from build123d import *

# Parameters (mm, degrees)
SKETCH1_R           = 32.5
BOSS_EXTRUDE1_DEPTH = 3
BOSS_EXTRUDE6_DEPTH = 3
CUT_EXTRUDE1_DEPTH  = 3
SKETCH5_R           = 7
BOSS_EXTRUDE7_DEPTH = 3
SKETCH7_R           = 1.9
CUT_EXTRUDE2_DEPTH  = 3


with BuildPart() as part:
    # Sketch1 → Boss-Extrude1 (new body)
    with BuildSketch(Plane.XY):
        Circle(SKETCH1_R)
    extrude(amount=BOSS_EXTRUDE1_DEPTH)

    # Sketch2 → Boss-Extrude6 (add)
    with BuildSketch(Plane.XY.offset(3)):
        Polygon((-0.480921932, 36), (-2.2, 32.425452965), (2.2, 32.425452965), (0.480921932, 36), align=None)
        Polygon((6.106641727, 35.481547496), (7.245372738, 31.682086009), (2.899544039, 32.370397655), (5.156639756, 35.632013027), align=None)
        Polygon((11.581995735, 34.089421537), (12.112340352, 30.158600949), (7.927691681, 31.518275724), (10.66722786, 34.386647637), align=None)
        Polygon((16.77216257, 31.857900882), (16.681061949, 27.892511042), (12.760633243, 29.890069241), (15.915153411, 32.294568859), align=None)
        Polygon((21.549343099, 28.841932978), (20.839040439, 24.939614944), (17.279365664, 27.525870054), (20.771195066, 29.407290617), align=None)
        Polygon((25.795907282, 25.115780963), (24.483892593, 21.372622756), (21.372622756, 24.483892593), (25.115780963, 25.795907282), align=None)
        Polygon((29.407290617, 20.771195066), (27.525870054, 17.279365664), (24.939614944, 20.83904044), (28.841932978, 21.549343099), align=None)
        Polygon((32.294568859, 15.915153411), (29.890069241, 12.760633243), (27.892511042, 16.681061949), (31.857900882, 16.77216257), align=None)
        Polygon((34.386647637, 10.66722786), (31.518275724, 7.927691681), (30.158600949, 12.112340352), (34.089421537, 11.581995735), align=None)
        Polygon((35.632013027, 5.156639756), (32.370397655, 2.899544039), (31.682086009, 7.245372738), (35.481547496, 6.106641727), align=None)
        Polygon((36, -0.480921932), (32.425452965, -2.2), (32.425452965, 2.2), (36, 0.480921932), align=None)
        Polygon((35.481547496, -6.106641727), (31.682086009, -7.245372738), (32.370397655, -2.899544039), (35.632013027, -5.156639756), align=None)
        Polygon((34.089421537, -11.581995735), (30.158600949, -12.112340352), (31.518275724, -7.927691681), (34.386647637, -10.66722786), align=None)
        Polygon((31.857900882, -16.77216257), (27.892511042, -16.681061949), (29.890069241, -12.760633243), (32.294568859, -15.915153411), align=None)
        Polygon((28.841932978, -21.549343099), (24.939614944, -20.839040439), (27.525870054, -17.279365664), (29.407290617, -20.771195066), align=None)
        Polygon((25.115780963, -25.795907282), (21.372622756, -24.483892593), (24.483892593, -21.372622756), (25.795907282, -25.115780963), align=None)
        Polygon((20.771195066, -29.407290617), (17.279365664, -27.525870054), (20.83904044, -24.939614944), (21.549343099, -28.841932978), align=None)
        Polygon((15.915153411, -32.294568859), (12.760633243, -29.890069241), (16.681061949, -27.892511042), (16.77216257, -31.857900882), align=None)
        Polygon((10.66722786, -34.386647637), (7.927691681, -31.518275724), (12.112340352, -30.158600949), (11.581995735, -34.089421537), align=None)
        Polygon((5.156639756, -35.632013027), (2.899544039, -32.370397655), (7.245372738, -31.682086009), (6.106641727, -35.481547496), align=None)
        Polygon((-0.480921932, -36), (-2.2, -32.425452965), (2.2, -32.425452965), (0.480921932, -36), align=None)
        Polygon((-6.106641727, -35.481547496), (-7.245372738, -31.682086009), (-2.899544039, -32.370397655), (-5.156639756, -35.632013027), align=None)
        Polygon((-11.581995735, -34.089421537), (-12.112340352, -30.158600949), (-7.927691681, -31.518275724), (-10.66722786, -34.386647637), align=None)
        Polygon((-16.77216257, -31.857900882), (-16.681061949, -27.892511042), (-12.760633243, -29.890069241), (-15.915153411, -32.294568859), align=None)
        Polygon((-21.549343099, -28.841932978), (-20.839040439, -24.939614944), (-17.279365664, -27.525870054), (-20.771195066, -29.407290617), align=None)
        Polygon((-25.795907282, -25.115780963), (-24.483892593, -21.372622756), (-21.372622756, -24.483892593), (-25.115780963, -25.795907282), align=None)
        Polygon((-29.407290617, -20.771195066), (-27.525870054, -17.279365664), (-24.939614944, -20.83904044), (-28.841932978, -21.549343099), align=None)
        Polygon((-32.294568859, -15.915153411), (-29.890069241, -12.760633243), (-27.892511042, -16.681061949), (-31.857900882, -16.77216257), align=None)
        Polygon((-34.386647637, -10.66722786), (-31.518275724, -7.927691681), (-30.158600949, -12.112340352), (-34.089421537, -11.581995735), align=None)
        Polygon((-35.632013027, -5.156639756), (-32.370397655, -2.899544039), (-31.682086009, -7.245372738), (-35.481547496, -6.106641727), align=None)
        Polygon((-36, 0.480921932), (-32.425452965, 2.2), (-32.425452965, -2.2), (-36, -0.480921932), align=None)
        Polygon((-35.481547496, 6.106641727), (-31.682086009, 7.245372738), (-32.370397655, 2.899544039), (-35.632013027, 5.156639756), align=None)
        Polygon((-34.089421537, 11.581995735), (-30.158600949, 12.112340352), (-31.518275724, 7.927691681), (-34.386647637, 10.66722786), align=None)
        Polygon((-31.857900882, 16.77216257), (-27.892511042, 16.681061949), (-29.890069241, 12.760633243), (-32.294568859, 15.915153411), align=None)
        Polygon((-28.841932978, 21.549343099), (-24.939614944, 20.839040439), (-27.525870054, 17.279365664), (-29.407290617, 20.771195066), align=None)
        Polygon((-25.115780963, 25.795907282), (-21.372622756, 24.483892593), (-24.483892593, 21.372622756), (-25.795907282, 25.115780963), align=None)
        Polygon((-20.771195066, 29.407290617), (-17.279365664, 27.525870054), (-20.839040439, 24.939614944), (-21.549343099, 28.841932978), align=None)
        Polygon((-15.915153411, 32.294568859), (-12.760633243, 29.890069241), (-16.681061949, 27.892511042), (-16.77216257, 31.857900882), align=None)
        Polygon((-10.66722786, 34.386647637), (-7.927691681, 31.518275724), (-12.112340352, 30.158600949), (-11.581995735, 34.089421537), align=None)
        Polygon((-5.156639756, 35.632013027), (-2.899544039, 32.370397655), (-7.245372738, 31.682086009), (-6.106641727, 35.481547496), align=None)
    extrude(amount=-BOSS_EXTRUDE6_DEPTH)

    # Sketch3 → Cut-Extrude1 (cut)
    with BuildSketch(Plane.XY.offset(3)):
        with BuildLine():
            Line((-2.337034435, 0.887845736), (-0.197962265, -2.492149863))
            ThreePointArc((-0.197962265, -2.492149863), (1.336920106, -2.11249725), (2.337034435, -0.887845736))
            Line((2.337034435, -0.887845736), (0.197962265, 2.492149863))
            ThreePointArc((0.197962265, 2.492149863), (-1.336920106, 2.11249725), (-2.337034435, 0.887845736))
        make_face()
    extrude(amount=-CUT_EXTRUDE1_DEPTH, mode=Mode.SUBTRACT)

    # Sketch5 → Boss-Extrude7 (add)
    with BuildSketch(Plane(origin=(0, 0, 0), x_dir=(-1, 0, 0), z_dir=(0, 0, -1))):
        with Locations(Location((0, 0, 0), (0, 0, 180))):
            Circle(SKETCH5_R)
        with BuildLine():
            Line((-0.197962265, 2.492149863), (-2.337034435, -0.887845736))
            ThreePointArc((-2.337034435, -0.887845736), (-1.336920106, -2.11249725), (0.197962265, -2.492149863))
            Line((0.197962265, -2.492149863), (2.337034435, 0.887845736))
            ThreePointArc((2.337034435, 0.887845736), (1.336920106, 2.11249725), (-0.197962265, 2.492149863))
        make_face(mode=Mode.SUBTRACT)
    extrude(amount=BOSS_EXTRUDE7_DEPTH)

    # Sketch7 → Cut-Extrude2 (cut)
    with BuildSketch(Plane.XY.offset(3)):
        with Locations((0, 22)):
            Circle(SKETCH7_R)
    extrude(amount=-CUT_EXTRUDE2_DEPTH, mode=Mode.SUBTRACT)


solid = part.part
Can you work these out from the model? Positions are in its coordinate system, mm. A direction names the side the tool comes from. Round coordinates to 2 decimals unless told otherwise and drop trailing zeros. Order: outer loops, then holes, each group sorted by start corner. A loop starts at its lowest first (then second) coordinate and runs counter-clockwise, first axis right, second up. Notation, with made-up numbers: M 78,36.25 L 125,36.25 A14 ccw 125,57.25 Z; hole C 45.25,40 d7. An arc over 180 degrees is marked long. Use a Markdown table: item, result.
1) I'm going to push flat-ended pins straight in: P1, Ø2, axis at x = -10, z = 1, coming from the +Y side; P2, Ø3.5, axis at x = 0, y = 22, coming from the +Z side. Where does each tip first touch, or does it pass through?
Geometry says:
| item | result |
|---|---|
| P1 | stops at y = 34.39 |
| P2 | passes through |
2) Imagine slicing it at C-C (x = -15). List the corners of the cut face in (y, z) for me, then the cut area to 3 significant figures.
Geometry says:
| item | result |
|---|---|
| outline | M -31.6,0 L 31.6,0 L 31.6,3 L -31.6,3 Z |
| area | 190 mm² |
3) Imagine slicing it at B-B (y = -9). List the corners of the cut face in (x, z) for me, then the cut area to 3 significant figures.
Geometry says:
| item | result |
|---|---|
| outline | M -32.64,0 L 32.64,0 L 32.64,3 L -32.64,3 Z |
| area | 196 mm² |
4) If we mould it in two halves opening along Y, with no side actions, what happens to faces 1 (the face through (-11.85, 32.1, 1.52)), 2 (the face through (-34.238, 1.328, 1.521)), 3 (the face through (6.466, 2.681, -1.479))? For each: +Y half, -Y half, draft (parallel to the pull), parting line (faces both ways), or undercut.
Geometry says:
| item | result |
|---|---|
| face 1 | +Y half |
| face 2 | undercut |
| face 3 | parting line |
5) Imagine slicing it at A-A (z = 2.05). Give the number of separate pieces and of enclosed holes in the cut face, then the cut area to 3 significant figures.
Geometry says:
| item | result |
|---|---|
| separate pieces | 1 |
| enclosed holes | 2 |
| area | 3,670 mm² |
6) If I drill on line 1 along Y through (x, z) = (0, 1.4); line 2 along Z through (x, y) = (-9.5, -6); line 3 along Y through (x, z) = (8, 0.3), over which ranges is the centre line in solid material (lowest first)?
Geometry says:
| item | result |
|---|---|
| line 1 | y = -36 to -2.5, 2.5 to 20.1, 23.9 to 36 |
| line 2 | z = 0 to 3 |
| line 3 | y = -31.59 to 31.59 |
7) On a 3-axis mill with a long thin cutter (end or side, diameter ignored), from which of +Z, -Z, +X, -X, +Y, -Y can I reach the whole of each face in a straight line? I mean faces 4 (the face through (34.02, 4.04, 1.52)), 5 (the face through (21.2, 26.92, 1.52)), 6 (the face through (-32.152, 11.843, 1.521)), 7 (the face through (-19.001, -28.453, 1.521)), 8 (the face through (-1.328, 34.238, 1.521)). Say none if no direction works.
Geometry says:
| item | result |
|---|---|
| face 4 | +Z, -Z, +X |
| face 5 | +Z, -Z |
| face 6 | +Z, -Z, -X |
| face 7 | +Z, -Z, -Y |
| face 8 | +Z, -Z, +Y |
